Source: CAD feature listing. Evaluate the final solid. Frame: model axes, mm. Face numbers are marked on the shaded views. Coordinates: 2 decimals unless noted, no trailing zeros. Loops run counter-clockwise (first coordinate to the right, second up) from the corner with the lowest first, then second, coordinate; pieces in that order, holes last. Notation, with made-up numbers: (65, 43) - (114, 43) arc R28 ccw to (114, 81) - close; hole circle Ø7 at (-22.5, 21). An arc over 180 degrees is marked (long way). Write item = value, one per line. Start each with the question number.
from build123d import *

# Parameters (mm, degrees)
F0_W         = 35
F0_H         = 35
F1_DEPTH     = 6.5
F2_R         = 2.125
F3_DEPTH     = 13.001
F4_R         = 5
F5_T1_DEPTH  = 25
F5_T3_DEPTH  = 25
F5_T12_ANGLE = 90
F5_T14_ANGLE = 90
F5_T16_ANGLE = 90
F5_T18_ANGLE = 90
F6_R         = 2.5
F7_DEPTH     = 13.001
F8_SIZE      = 1


# Not quite as in the source:
# - a fillet or chamfer that OpenCascade refuses, or shapes differently, is made with other operations: its cross-section is extruded or revolved along the edge and cut away or added


with BuildPart() as f1:
    # F0 (on Top) → F1 (new body, symmetric)
    with BuildSketch(Plane.XY):
        Rectangle(F0_W, F0_H)
    extrude(amount=F1_DEPTH, both=True)

    # F2 (on face) → F3 (cut, through all)
    with BuildSketch(Plane.XY.offset(6.5)):
        with Locations((-12.5, -12.9)):
            Circle(F2_R)
        with Locations((-12.5, 12.5)):
            Circle(F2_R)
        with Locations((12.5, 12.5)):
            Circle(F2_R)
        with Locations((12.5, -12.9)):
            Circle(F2_R)
    extrude(amount=-F3_DEPTH, mode=Mode.SUBTRACT)

    # F4
    f4_edges = [f1.edges().sort_by_distance(p)[0] for p in [
        (-17.5, 17.5, 0),
        (17.5, 17.5, 0),
        (17.5, -17.5, 0),
        (-17.5, -17.5, 0),
    ]]
    fillet(f4_edges, radius=F4_R)

    # F5: chamfer of 1.4 x 2.8 on 12 edges, made by hand

    # F5_s2 → F5_t1 (cut)
    with BuildSketch(Plane.XZ.offset(-12.5)):
        Polygon((17.5, -3.7), (16.1, -6.5), (17.5, -6.5), align=None)
        Polygon((-16.1, -6.5), (-17.5, -3.7), (-17.5, -6.5), align=None)
    extrude(amount=F5_T1_DEPTH, mode=Mode.SUBTRACT)

    # F5_s4 → F5_t3 (cut)
    with BuildSketch(Plane.YZ.offset(-12.5)):
        Polygon((-16.1, -6.5), (-17.5, -3.7), (-17.5, -6.5), align=None)
        Polygon((16.1, -6.5), (17.5, -3.7), (17.5, -6.5), align=None)
    extrude(amount=F5_T3_DEPTH, mode=Mode.SUBTRACT)

    # F5_s5 → F5_t6 (revolve, cut)
    with BuildSketch(Plane.XZ.offset(12.9)):
        Polygon((-8.975, -6.5), (-10.375, -3.7), (-10.375, -6.5), align=None)
    revolve(axis=Axis((-12.5, -12.9, -6.5), (0, 0, 1)), mode=Mode.SUBTRACT)

    # F5_s7 → F5_t8 (revolve, cut)
    with BuildSketch(Plane.XZ.offset(12.9)):
        Polygon((16.025, -6.5), (14.625, -3.7), (14.625, -6.5), align=None)
    revolve(axis=Axis((12.5, -12.9, -6.5), (0, 0, 1)), mode=Mode.SUBTRACT)

    # F5_s9 → F5_t10 (revolve, cut)
    with BuildSketch(Plane.XZ.offset(-12.5)):
        Polygon((16.025, -6.5), (14.625, -3.7), (14.625, -6.5), align=None)
    revolve(axis=Axis((12.5, 12.5, -6.5), (0, 0, 1)), mode=Mode.SUBTRACT)

    # F5_s11 → F5_t12 (revolve, cut)
    with BuildSketch(Plane.XZ.offset(12.5)):
        Polygon((16.1, -6.5), (17.5, -3.7), (17.5, -6.5), align=None)
    revolve(axis=Axis((12.5, -12.5, -6.5), (0, 0, -1)), revolution_arc=F5_T12_ANGLE, mode=Mode.SUBTRACT)

    # F5_s13 → F5_t14 (revolve, cut)
    with BuildSketch(Plane.XZ.offset(-12.5)):
        Polygon((16.1, -6.5), (17.5, -3.7), (17.5, -6.5), align=None)
    revolve(axis=Axis((12.5, 12.5, -6.5), (0, 0, 1)), revolution_arc=F5_T14_ANGLE, mode=Mode.SUBTRACT)

    # F5_s15 → F5_t16 (revolve, cut)
    with BuildSketch(Plane.YZ.offset(-12.5)):
        Polygon((-16.1, -6.5), (-17.5, -3.7), (-17.5, -6.5), align=None)
    revolve(axis=Axis((-12.5, -12.5, -6.5), (0, 0, -1)), revolution_arc=F5_T16_ANGLE, mode=Mode.SUBTRACT)

    # F5_s17 → F5_t18 (revolve, cut)
    with BuildSketch(Plane.YZ.offset(-12.5)):
        Polygon((16.1, -6.5), (17.5, -3.7), (17.5, -6.5), align=None)
    revolve(axis=Axis((-12.5, 12.5, -6.5), (0, 0, 1)), revolution_arc=F5_T18_ANGLE, mode=Mode.SUBTRACT)

    # F5_s19 → F5_t20 (revolve, cut)
    with BuildSketch(Plane.XZ.offset(-12.5)):
        Polygon((-8.975, -6.5), (-10.375, -3.7), (-10.375, -6.5), align=None)
    revolve(axis=Axis((-12.5, 12.5, -6.5), (0, 0, 1)), mode=Mode.SUBTRACT)

    # F6 (on face) → F7 (cut, through all)
    with BuildSketch(Plane(origin=(0, 0, -6.5), x_dir=(1, 0, 0), z_dir=(0, 0, -1))):
        Circle(F6_R)
    extrude(amount=-F7_DEPTH, mode=Mode.SUBTRACT)

    # F8
    f8_edges = [f1.edges().sort_by_distance(p)[0] for p in [
        (-17.5, 0, 6.5),
    ]]
    chamfer(f8_edges, length=F8_SIZE)


solid = f1.part
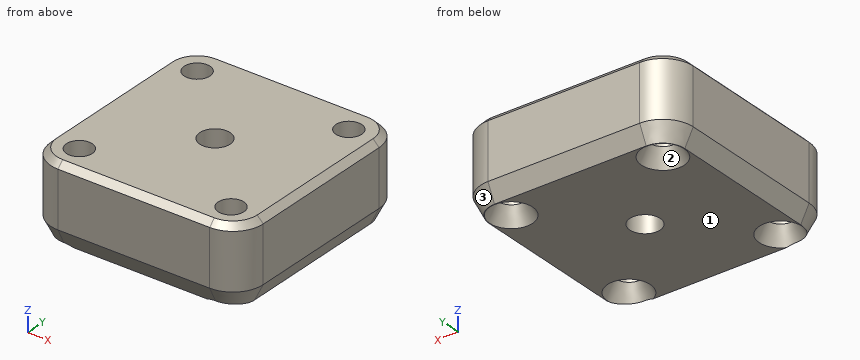
Item 1: First-contact query: pin 1 (6 mm diameter, centred on x = 0, y = 0, fed in from -Z). Flat tip, straight axial feed; report the tip coordinate or a pass-through.
Item 2: Cut plane A-A (z = 4.5). Return the cut outline in (x, y) (3 decimals), then the cut area to 3 significant figures.
Item 3: Cut plane B-B (y = 0). Return the cut outline in (x, z).
Item 4: Cut plane D-D (y = 12). State how many separate pieces and enclosed holes the cut face has, then the cut area to 3 significant figures.
Item 5: Draft query along X for the marked faces 1, 2 and 3. Return one class per face: released by +X, released by -X, zero draft, split by the parting line, or undercut.
Item 6: Material intervals for L1, parallel to Y at x = 12.5, z = 0.5 (3 decimals); L2, parallel to Y at x = 0, z = 2.5; L3, parallel to Y at x = 11, z = -2.5, sorted ascending. Write a range as [from, to].
Responses:
q1.pin_1 = -6.5
q2.outline = (-17.5, -12.5) arc R5 ccw to (-12.5, -17.5) - (12.5, -17.5) arc R5 ccw to (17.5, -12.5) - (17.5, 12.5) arc R5 ccw to (12.5, 17.5) - (-12.5, 17.5) arc R5 ccw to (-17.5, 12.5) - close; hole circle Ø4.25 at (-12.5, -12.9); hole circle Ø4.25 at (-12.5, 12.5); hole circle Ø5 at (0, 0); hole circle Ø4.25 at (12.5, -12.9); hole circle Ø4.25 at (12.5, 12.5)
q2.area = 1,130 mm2
q3.outline = (-17.5, -3.7) - (-16.1, -6.5) - (-2.5, -6.5) - (-2.5, 6.5) - (-16.5, 6.5) - (-17.5, 5.5) - close; (2.5, -6.5) - (16.1, -6.5) - (17.5, -3.7) - (17.5, 5.5) - (16.5, 6.5) - (2.5, 6.5) - close
q4.separate_pieces = 3
q4.enclosed_holes = 0
q4.area = 335 mm2
q5.face_1 = zero draft
q5.face_2 = undercut
q5.face_3 = released by +X
q6.L1 = [-17.5, -15.025], [-10.775, 10.375], [14.625, 17.5]
q6.L2 = [-17.5, -2.5], [2.5, 17.5]
q6.L3 = [-17.5, -14.41], [-11.39, 10.99], [14.01, 17.5]
